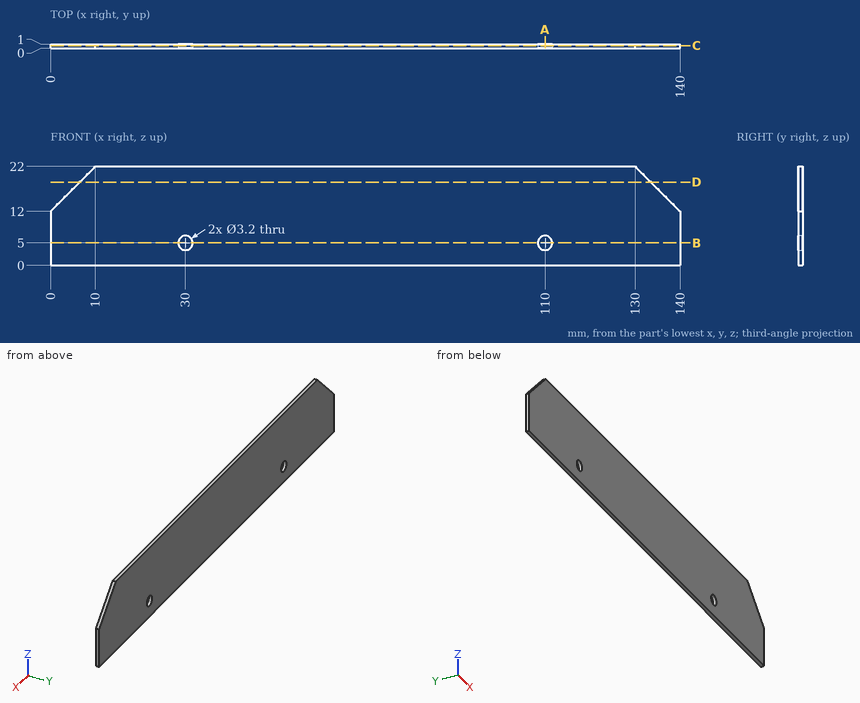
Can you work these out from the drawing? Everything is in mm from the part's minimum corner. Give positions to 0.01 mm unless a question says otherwise; leave off trailing zeros. Loops run counter-clockwise (first coordinate to the right, second up) from the corner with the lowest first, then second, coordinate; pieces in that order, holes last. Notation, with made-up numbers: M 48.25,74.25 L 68.25,74.25 A17 cw 68.25,103.25 Z; hole C 70.5,-21 d6. An arc over 180 degrees is marked long. Put each result on its own line as item: value. Start each with the question number.
(1) I want a section at B-B on z = 5. Please give me the cut outline in (x, y).
(2) Will this pin go through, and if not, where does the flat tip stop? pin 1 Ø2.5 at (x, z) = (110, 5) entering from +Y.
(3) I want a section at A-A on x = 110. Please give me the cut outline in (y, z), then the cut area to 3 significant figures.
(4) I need wall thicknesses on line 1 along X through (y, z) = (0.55, 5); line 2 along Z through (x, y) = (30, 0.55); line 3 along X through (y, z) = (0.1, 18.5). Which ranges of each line are inside material? Lowest first, please. Write a range as [from, to].
(5) I want a section at D-D on z = 18.5. Please give me the cut outline in (x, y), then the cut area to 3 significant figures.
(6) I want a section at C-C on y = 0.65. Please give me the cut outline in (x, z).
Answer block:
1. outline: M 0,0 L 28.4,0 L 28.4,1 L 0,1 Z; M 31.6,0 L 108.4,0 L 108.4,1 L 31.6,1 Z; M 111.6,0 L 140,0 L 140,1 L 111.6,1 Z
2. pin 1: through
3. outline: M 0,0 L 1,0 L 1,3.4 L 0,3.4 Z; M 0,6.6 L 1,6.6 L 1,22 L 0,22 Z
3. area: 18.8 mm^2
4. line 1: [0, 28.4], [31.6, 108.4], [111.6, 140]
4. line 2: [0, 3.4], [6.6, 22]
4. line 3: [6.5, 133.5]
5. outline: M 6.5,0 L 133.5,0 L 133.5,1 L 6.5,1 Z
5. area: 127 mm^2
6. outline: M 0,0 L 140,0 L 140,12 L 130,22 L 10,22 L 0,12 Z; hole C 30,5 d3.2; hole C 110,5 d3.2
